```python
from build123d import *

# Parameters (mm, degrees)
SKETCH2_W           = 200
SKETCH2_H           = 100
BOSS_EXTRUDE1_DEPTH = 1050
BOSS_EXTRUDE1_TAPER = 1
SHELL1_T            = -10


with BuildPart() as part:
    # Sketch2 → Boss-Extrude1 (new body)
    with BuildSketch(Plane.XY):
        Rectangle(SKETCH2_W, SKETCH2_H)
    extrude(amount=BOSS_EXTRUDE1_DEPTH, taper=BOSS_EXTRUDE1_TAPER)

    # Shell1
    shell1_openings = [part.faces().sort_by_distance(p)[0] for p in [
        (0, 0, 1050),
        (0, 0, 0),
    ]]
    offset(amount=SHELL1_T, openings=shell1_openings, kind=Kind.INTERSECTION)


solid = part.part
```
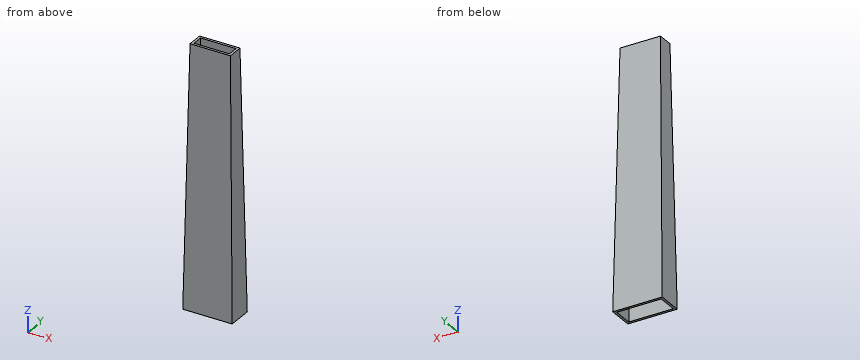
Verification items for the finished model (mm, model axes). Round coordinates to 2 decimals unless told otherwise and drop trailing zeros. Order: outer loops, then holes, each group sorted by start corner. A loop starts at its lowest first (then second) coordinate and runs counter-clockwise, first axis right, second up. Notation, with made-up numbers: (-6.75, 69.25) - (35.25, 69.25) arc R25 cw to (35.25, 95.25) - close; hole circle Ø10 at (-27, 36). An arc over 180 degrees is marked (long way). Use CSV: the item, a comma, the result in double quotes. Start each with the question number.
1) Go/stop test with flat-tipped pins: P1, Ø12, axis at y = 24, z = 115, coming from the +X side; P2, Ø1.5, axis at x = 52.5, z = 686.5, coming from the -Y side; P3, Ø8, axis at x = -76.5, z = 223, coming from the -Y side. Record where each tip stops, or that it passes through.
2) Thickness scan on L1, parallel to X at y = -10, z = 320.5; L2, parallel to X at y = 22.5, z = 395.5 (3 decimals); L3, parallel to Y at x = -9, z = 965. Record the ranges inside material, lowest first.
3) Section check B-B, the plane x = -19.5. Record the cut outline in (y, z), plus the area to 3 significant figures.
4) Section check C-C, the plane z = 83. Record the cut outline in (x, y).
5) Section check D-D, the plane z = 655. Record the cut outline in (x, y), plus the area to 3 significant figures.
6) Section check A-A, the plane y = 6.5. Record the cut outline in (x, z), plus the area to 3 significant figures.
Answers:
1,P1,"stops at x = 98.1"
1,P2,"stops at y = -38.03"
1,P3,"stops at y = -46.18"
2,L1,"x = -94.41 to -84.4, 84.4 to 94.41"
2,L2,"x = -93.097 to -83.095, 83.095 to 93.097"
2,L3,"y = -33.16 to -23.15, 23.15 to 33.16"
3,outline,"(-50, 0) - (-40, 0) - (-21.67, 1050) - (-31.67, 1050) - close; (21.67, 1050) - (40, 0) - (50, 0) - (31.67, 1050) - close"
3,area,"21,000 mm²"
4,outline,"(-98.55, -48.55) - (98.55, -48.55) - (98.55, 48.55) - (-98.55, 48.55) - close; hole (-88.55, -38.55) - (88.55, -38.55) - (88.55, 38.55) - (-88.55, 38.55) - close"
5,outline,"(-88.57, -38.57) - (88.57, -38.57) - (88.57, 38.57) - (-88.57, 38.57) - close; hole (-78.57, -28.57) - (78.57, -28.57) - (78.57, 28.57) - (-78.57, 28.57) - close"
5,area,"4,690 mm²"
6,outline,"(-100, 0) - (-90, 0) - (-71.67, 1050) - (-81.67, 1050) - close; (71.67, 1050) - (90, 0) - (100, 0) - (81.67, 1050) - close"
6,area,"21,000 mm²"
